Build history of the part. All positions in model axes, mm. A direction names the side the tool comes from. Round coordinates to 2 decimals unless told otherwise and drop trailing zeros. Answer as a JSON object with one key per item and string values. Group by question number.
Item 1: Slice it at A-A, the plane y = 5.4. Give the number of separate pieces and of enclosed holes in the cut face, then the cut area to 3 significant figures.
Item 2: Probe line 1 (Y direction, x = -2, z = -12); line 2 (Y direction, x = -2.7, z = 0); line 3 (Y direction, x = -2.2, z = 0). List the from-to ranges inside material, lowest first. Write a range as from..to.
Item 3: Flat gauge pins, fed straight in: pin 1 (3.5 mm diameter, centred on y = 5.5, z = 7, fed in from -X); pin 2 (2 mm diameter, centred on x = -1, z = -8, fed in from +Y); pin 3 (2 mm diameter, centred on x = 15.5, z = 3, fed in from +Y); pin 4 (0.6 mm diameter, centred on x = -1.5, z = -10.5, fed in from -Y). Where does each tip first touch, or does it go through?
Item 4: Two-plate mould, pull along Y, no slides. Class faces 5 (the flat face through (7, 19, -2.1)), 6 (the cylindrical face through (-2.218, 4.521, 0.195)), 7 (the flat face through (8.855, 17.658, 11.713)): +Y half, -Y half, draft (parallel to the pull), parting line (faces both ways), or undercut.
Item 5: Which spindle directions (+Z, -Z, +X, -X, +Y, -Y) get a long thin tool onto all of the face, cutting with end or side? Do faces 1 (the flat face through (7, 16, 4)), 2 (the flat face through (14.5, 8, 13)), 3 (the flat face through (7, 12.3, 0)), 4 (the flat face through (11.25, 19, 0)). Say none if no direction does.
Autodesk Inventor part; units mm, degrees
ref_plane "Work Plane1" through (10.75, 0, 0) normal (1, 0, 0) x (0, 1, 0)
ref_plane "XZ Plane" through (0, 0, 0) normal (0, 1, 0) x (-1, 0, 0)
ref_plane "XY Plane" through (0, 0, 0) normal (0, 0, 1) x (1, 0, 0)
sketch "Sketch1" plane through (0, 0, 0) normal (0, 0, 1) x (1, 0, 0)
  line L0 (0, 0) -> (0, 12.3)
  line L1 (0, 12.3) -> (14.5, 12.3)
  line L2 (14.5, 12.3) -> (14.5, 0)
  line L3 (14.5, 0) -> (19, 0)
  line L4 (19, 0) -> (19, 14.3)
  line L5 (19, 14.3) -> (-4.5, 14.3)
  line L6 (-4.5, 14.3) -> (-4.5, 0)
  line L7 (-4.5, 0) -> (0, 0)
  dimension "d6" = 12.3
  dimension "d7" = 14.5
  dimension "d8" = 4.5
  dimension "d9" = 14.3
  dimension "d10" = 23.5
  dimension "d108" = 12.3
  dimension "d205" = 4.5
extrude "Extrusion1" add sketch "Sketch1" along normal mid plane 10
sketch "Sketch2" plane through (-4.5, 14.3, 5) normal (0, 1, 0) x (1, 0, 0)
  line L0 (0, 10) -> (0, 0)
  line L1 (0, 10) -> (23.5, 10)
  line L2 (0, 0) -> (23.5, 10)
  line L3 (23.5, 0) -> (0, 0)
  line L4 (0, 10) -> (23.5, 0)
  line L5 (9.65, 2.9) -> (13.85, 2.9)
  line L6 (13.85, 2.9) -> (13.85, 7.1)
  line L7 (13.85, 7.1) -> (9.65, 7.1)
  line L8 (9.65, 7.1) -> (9.65, 2.9)
  line L9 (9.65, 2.9) -> (13.85, 7.1) construction
  line L10 (13.85, 2.9) -> (9.65, 7.1) construction
  line L11 (7.75, 1) -> (15.75, 1)
  line L12 (15.75, 1) -> (15.75, 9)
  line L13 (15.75, 9) -> (7.75, 9)
  line L14 (7.75, 9) -> (7.75, 1)
  line L15 (7.75, 1) -> (15.75, 9) construction
  line L16 (15.75, 1) -> (7.75, 9) construction
  point P0 (4.5, 5)
  point P1 (11.75, 5)
  dimension "d11" = 4.2
  dimension "d12" = 4.2
  dimension "d13" = 8
  dimension "d14" = 8
extrude "Extrusion2" add sketch "Sketch2" along normal blind 10 contours L14 L13 L12 L2 L6 L7 L8 L4 | L4 L8 L2 L14 | L2 L8 L5 L6 L4 L12 L11 L14 | L12 L4 L6 L2
sketch "Sketch3" plane through (0, 0, 5) normal (1, 0, 0) x (0, 0, -1)
  line L0 (10, 0) -> (0, 0)
  line L1 (0, 0) -> (5, 0)
  line L2 (10, 14.3) -> (0, 14.3)
  line L3 (6.95, 14.3) -> (3.05, 14.3)
  line L4 (5, 0) -> (5, 2)
  line L5 (8.4, 5.4) -> (17.767, 5.4) construction
  line L6 (6.8, 5.4) -> (16.167, 5.4) construction
  line L7 (1.6, 5.4) -> (10.967, 5.4) construction
  line L8 (3.2, 5.4) -> (12.567, 5.4) construction
  line L9 (5, 5.4) -> (5, 0)
  line L10 (5, 8.8) -> (5, 10.4)
  line L11 (5, 10.4) -> (19, 10.4)
  line L12 (5, 0) -> (19, 0)
  line L13 (19, 0) -> (19, 10.4)
  line L14 (5, 8.8) -> (5, 0)
  point P0 (1.9, 14.3)
  point P1 (8.1, 14.3)
  point P2 (10, 0)
  dimension "d17" = 5
  dimension "d111" = 2
  dimension "d172" = 1.6
  dimension "d173" = 14
  dimension "d174" = 14
extrude "Extrusion3" add sketch "Sketch3" against normal blind 4.5
ref_plane "Work Plane1" through (10.75, 0, 0) normal (1, 0, 0) x (0, 1, 0)
sketch "Sketch15" plane through (10.75, 0, 0) normal (1, 0, 0) x (0, 1, 0)
  line L0 (24.3, -4) -> (24.3, 4)
  line L1 (24.3, 4) -> (19.3, 12.6603)
  line L2 (24.3, 4) -> (34.3, 4) construction
  line L3 (24.3, 4) -> (16.3, 4)
  line L4 (14.3, 4) -> (24.3, 4)
  line L5 (19.3, 12.6603) -> (13.2378, 9.1603)
  line L6 (13.2378, 9.1603) -> (16.2171, 4)
  line L7 (13.2378, 9.1603) -> (19.1964, 9.1603) construction
  point P0 (0, 0)
  point P1 (18.5265, 4)
  dimension "d83" = 10
  dimension "d84" = 120
  dimension "d85" = 8
  dimension "d93" = 7
  dimension "d94" = 60
extrude "Extrusion13" add sketch "Sketch15" against normal blind 7
sketch "Sketch17" plane through (3.75, 19.3, 12.6603) normal (0, -0.5, 0.866) x (1, 0, 0)
  line L0 (7, -7) -> (0, -7)
  line L1 (0, 0) -> (3.5, 0)
  line L2 (3.5, 0) -> (3.5, -3.5)
  circle A0 centre (3.5, -3.5) radius 2.1
  point P0 (-3.75, -23.0444)
  point P1 (0.25, -7)
  point P2 (6.5, -7)
  dimension "d119" = 3.5
  dimension "d120" = 3.5
  dimension "d121" = 4.2
extrude "Extrusion15" cut sketch "Sketch17" against normal blind 13
sketch "Sketch22" plane through (14.5, 0, 5) normal (-1, 0, 0) x (0, 0, 1)
  line L0 (-10, 0) -> (0, 0)
  line L1 (0, 0) -> (-5, 0)
  line L2 (-5, 0) -> (0.4, 0) construction
  line L3 (9, 8.8) -> (9, 0)
  line L4 (9, 0) -> (-5, 0)
  line L5 (9, 9.4295) -> (9, 0)
  line L6 (-5, 10.4) -> (9, 10.4)
  line L7 (9, 10.4) -> (9, 9.4295)
  line L8 (-5, 10.4) -> (-5, 0)
  point P0 (0, 0)
extrude "Extrusion20" add sketch "Sketch22" against normal blind 4.5
sketch "Sketch23" plane through (14.5, 0, -5) normal (-1, 0, 0) x (0, 0, 1)
  line L0 (0, 14.3) -> (0, 0)
  line L1 (0, 0) -> (5, 0)
  line L2 (0, 0) -> (19, 0)
  line L3 (5, 0) -> (5, 5.4)
  circle A0 centre (5, 5.4) radius 1.55
  circle A1 centre (5, 5.4) radius 3.4
  line L4 (5, 2) -> (20, 2)
  line L5 (5, 3.85) -> (20, 3.85)
  line L6 (5, 6.95) -> (20, 6.95)
  line L7 (5, 8.8) -> (20, 8.8)
  line L8 (20, 8.8) -> (20, 6.95)
  line L9 (20, 3.85) -> (20, 2)
  point P0 (8.0261, 3.85)
  point P1 (8.0261, 6.95)
  dimension "d161" = 5.4
  dimension "d162" = 3.1
  dimension "d163" = 6.8
  dimension "d164" = 15
  dimension "d165" = 15
  dimension "d166" = 15
extrude "Extrusion21" cut sketch "Sketch23" against normal blind 2.5 contours A1 L6 A0 L3 | L3 L5 A1 | A1 L5 L9 L4 | A0 L6 A1 L5 | L7 L8 L6 A1
sketch "Sketch24" plane through (14.5, 5.4, 0) normal (-1, 0, 0) x (0, 0, 1)
  circle A0 centre (0, 0) radius 0.9
  point P0 (0, -5.4)
  dimension "d169" = 1.8
extrude "Extrusion22" cut sketch "Sketch24" against normal through all
sketch "Sketch25" plane through (0, 0, 5) normal (1, 0, 0) x (0, 0, -1)
  line L0 (19, 0) -> (0, 0)
  line L1 (0, 0) -> (5, 0)
  line L2 (5, 0) -> (5, 5.4)
  line L3 (5, 0) -> (10.4, 0) construction
  circle A0 centre (5, 5.4) radius 1.55
  circle A1 centre (5, 5.4) radius 3.4
  line L4 (5, 8.8) -> (20, 8.8)
  line L5 (5, 6.95) -> (20, 6.95)
  line L6 (5, 3.85) -> (20, 3.85)
  line L7 (5, 2) -> (20, 2)
  line L8 (20, 2) -> (20, 3.85)
  line L9 (20, 6.95) -> (20, 8.8)
  point P0 (8.0261, 6.95)
  point P1 (8.0261, 3.85)
  dimension "d175" = 5.4
  dimension "d176" = 90
  dimension "d177" = 3.1
  dimension "d178" = 6.8
  dimension "d179" = 15
  dimension "d180" = 15
  dimension "d181" = 15
  dimension "d182" = 15
extrude "Extrusion23" cut sketch "Sketch25" against normal blind 2.5 contours A1 L5 A0 L2 | L2 L6 A1 | A1 L6 L8 L7 | A0 L5 A1 L6 | L4 L9 L5 A1
sketch "Sketch26" plane through (0, 5.4, 0) normal (1, 0, 0) x (0, 0, -1)
  circle A0 centre (0, 0) radius 0.9
  point P0 (0, -5.4)
  dimension "d185" = 1.8
extrude "Extrusion24" cut sketch "Sketch26" against normal through all
sketch "Sketch27" plane through (0, 5.4, 0) normal (1, 0, 0) x (0, 0, -1)
  circle A0 centre (0, 0) radius 0.9
  arc A1 (-5, -2.0396) -> (0, -5.4) centre (0, 0) ccw
  line L0 (-5, 8.9) -> (-5, -5.4)
  line L1 (-5, -2.0396) -> (-5, -5.4)
  line L2 (-5, -5.4) -> (0, -5.4)
extrude "Extrusion25" cut sketch "Sketch27" against normal through all contours A1 L2 L0
sketch "Sketch28" plane through (14.5, 5.4, 0) normal (-1, 0, 0) x (0, 0, 1)
  arc A0 (-5, -2.0388) -> (0.0007, -5.4) centre (0.0003, 0) ccw
  line L0 (-5, 8.9) -> (-5, -5.4)
  line L1 (-5, -2.0388) -> (-5, -5.4)
  line L2 (-5, -5.4) -> (0, -5.4)
extrude "Extrusion26" cut sketch "Sketch28" against normal through all
fillet "Fillet9" radius 0.5 12 edges at (17, 8.8, 7) (17, 2, 7) (17, 5.4, -3.4) (17, 5.4, -1.55) (17, 6.95, 8.5131) (17, 3.85, 8.5131) (-2.5, 8.8, -7) (-2.5, 2, -7) (-2.5, 5.4, 3.4) (-2.5, 6.95, -8.5131) (-2.5, 3.85, -8.5131) (-2.5, 5.4, 1.55)
sketch "Sketch29" plane through (0, 3.85, -14) normal (1, 0, 0) x (0, 0, -1)
  line L0 (0, 6.55) -> (0, -3.85)
  line L1 (0, -3.85) -> (-2, -3.85)
  line L2 (0, -3.85) -> (-14, -3.85)
  line L3 (-2, -3.85) -> (-2, 6.55)
  line L4 (-9, 6.55) -> (0, 6.55)
  line L5 (-2, 6.55) -> (0, 6.55)
  line L6 (0, -3.85) -> (0, 6.55)
  dimension "d193" = 2
extrude "Extrusion27" add sketch "Sketch29" along normal blind 2
sketch "Sketch30" plane through (14.5, 3.85, 14) normal (-1, 0, 0) x (0, 0, 1)
  line L0 (0, 6.55) -> (0, -3.85)
  line L1 (0, -3.85) -> (-2, -3.85)
  line L2 (-14, -3.85) -> (0, -3.85)
  line L3 (-2, -3.85) -> (-2, 6.55)
  line L4 (-9, 6.55) -> (0, 6.55)
  line L5 (0, 6.55) -> (0, -3.85)
  dimension "d196" = 2
extrude "Extrusion28" add sketch "Sketch30" along normal blind 2
fillet "Fillet10" radius 1 4 edges at (12.5, 5.2, 14) (12.5, 5.2, 12) (2, 5.2, -12) (2, 5.2, -14)
sketch "Sketch31" plane through (3.75, 24.3, 4) normal (0, 0.866, 0.5) x (1, 0, 0)
  line L0 (-0.5, 0) -> (7, 0)
  line L1 (0, 0) -> (3.5, 0)
  line L2 (-0.5, 0) -> (7.5, 0)
  line L3 (3.5, 0) -> (3.5, -4)
  circle A0 centre (3.5, -4) radius 1.75
  point P0 (-3.75, -8.6859)
  dimension "d200" = 3.5
  dimension "d201" = 4
  dimension "d202" = 3.5
extrude "Extrusion29" cut sketch "Sketch31" against normal blind 2
properties part number "øvre del av kne Andre versjon"
Geometry says:
{
 "1": {"separate pieces": "4", "enclosed holes": "0", "area": "144 mm^2"},
 "2": {"line 1": "y = 0..2, 3.85..6.95, 8.8..10.4", "line 2": "y = 0..4.5, 6.3..14.3", "line 3": "y = 0..2.04, 3.81..4.5, 6.3..6.99, 8.76..14.3"},
 "3": {"pin 1": "stops at x = 14.5", "pin 2": "stops at y = 10.4", "pin 3": "stops at y = 14.3", "pin 4": "stops at y = 0"},
 "4": {"face 5": "draft", "face 6": "undercut", "face 7": "-Y half"},
 "5": {"face 1": "none", "face 2": "+Z", "face 3": "+Z, -Z, -Y", "face 4": "+Z, -Z, +X, +Y"}
}
